Check sheet for the drawn part. Datum: minimum x, y, z corner. Units: mm. Give positions to 0.01 mm unless a question says otherwise; leave off trailing zeros. Write each loop counter-clockwise with the first axis right and the second up, starting at its lowest first coordinate (ties: lowest second). Pieces come first, ordered by that corner, then holes. Notation, with made-up numbers: (-36.5, 32.5) - (17.5, 32.5) arc R28 ccw to (17.5, 66.5) - close; hole circle Ø10 at (29, -7.75). An arc over 180 degrees is marked (long way). One line per question, with ' | ' between items. Start each with the question number.
Q1. Section check B-B on y = 19.05. Record the boundary of the cut face in (x, z) (1 decimal).
Q2. Section check A-A on z = 11.5. Count the separate pieces of the cut face and the enclosed holes in it.
Q3. Gauge pin test, flat ends, axial feed: P1, Ø4, axis at y = 15, z = 32.5, coming from the +X side; P2, Ø11, axis at y = 26, z = 10.5, coming from the -X side (1 decimal); P3, Ø8, axis at y = 29, z = 44.5, coming from the +X side. Record the tip position at first contact, or that the pin passes through.
Q4. Section check C-C on z = 45.5. Record the boundary of the cut face in (x, y), and give its area (3 significant figures).
Q5. Thickness scan on L1, parallel to X at y = 32, z = 21 (1 decimal); L2, parallel to X at y = 36, z = 7.5 (1 decimal); L3, parallel to X at y = 15.5, z = 24 (1 decimal). Record the ranges inside material, lowest first. Write a range as [from, to].
Q6. Release check for a two-part mould opening along X. For the marked faces 1, 2 and 3 record: +X half, -X half, draft (parallel to the pull), parting line (faces both ways), or undercut.
Q7. Section check D-D on x = 5. Record the boundary of the cut face in (y, z) (1 decimal).
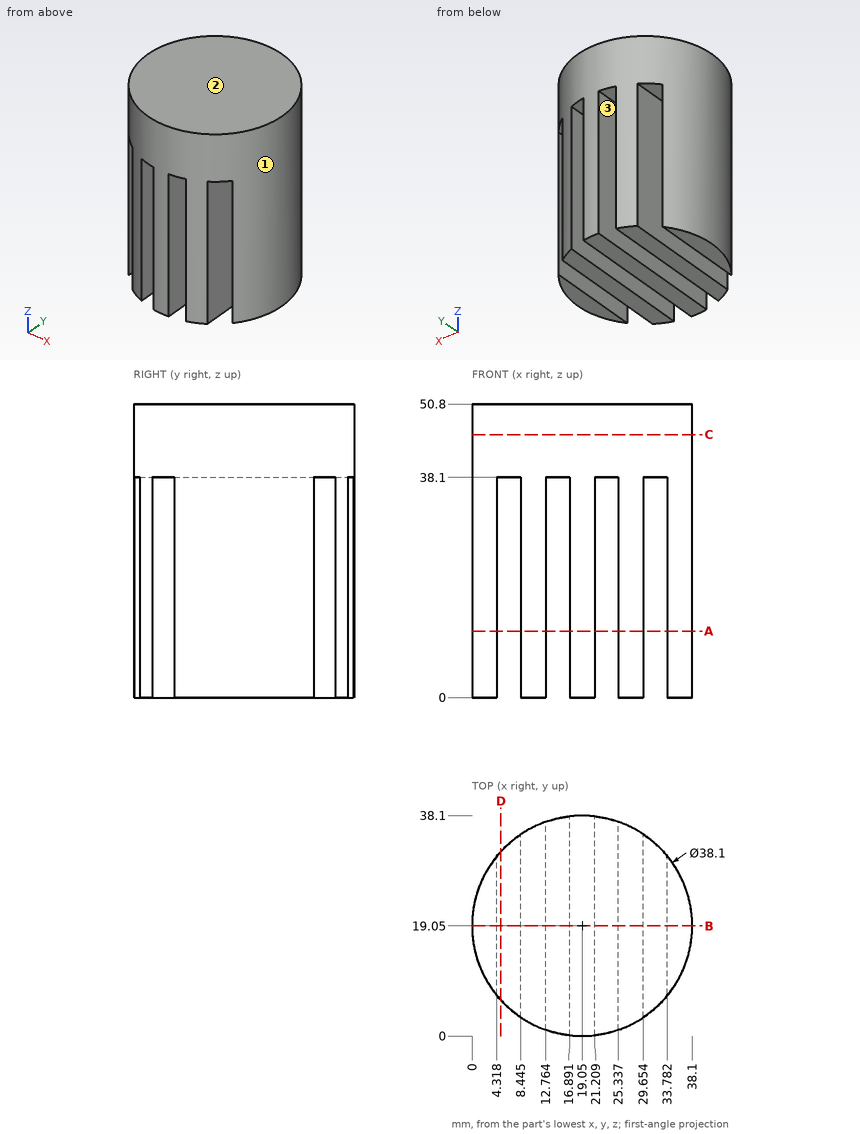
Working result:
1) outline: (0, 0) - (4.3, 0) - (4.3, 38.1) - (8.4, 38.1) - (8.4, 0) - (12.8, 0) - (12.8, 38.1) - (16.9, 38.1) - (16.9, 0) - (21.2, 0) - (21.2, 38.1) - (25.3, 38.1) - (25.3, 0) - (29.7, 0) - (29.7, 38.1) - (33.8, 38.1) - (33.8, 0) - (38.1, 0) - (38.1, 50.8) - (0, 50.8) - close
2) separate pieces: 5 | enclosed holes: 0
3) P1: stops at x = 37.99 | P2: stops at x = 0.1 | P3: stops at x = 37.15
4) outline: circle Ø38.1 at (19.05, 19.05) | area: 1,140 mm2
5) L1: x = [8.4, 12.8], [16.9, 21.2], [25.3, 29.7] | L2: x = [10.4, 12.8], [16.9, 21.2], [25.3, 27.7] | L3: x = [0.3, 4.3], [8.4, 12.8], [16.9, 21.2], [25.3, 29.7], [33.8, 37.8]
6) face 1: parting line | face 2: draft | face 3: undercut
7) outline: (6.2, 38.1) - (31.9, 38.1) - (31.9, 50.8) - (6.2, 50.8) - close
